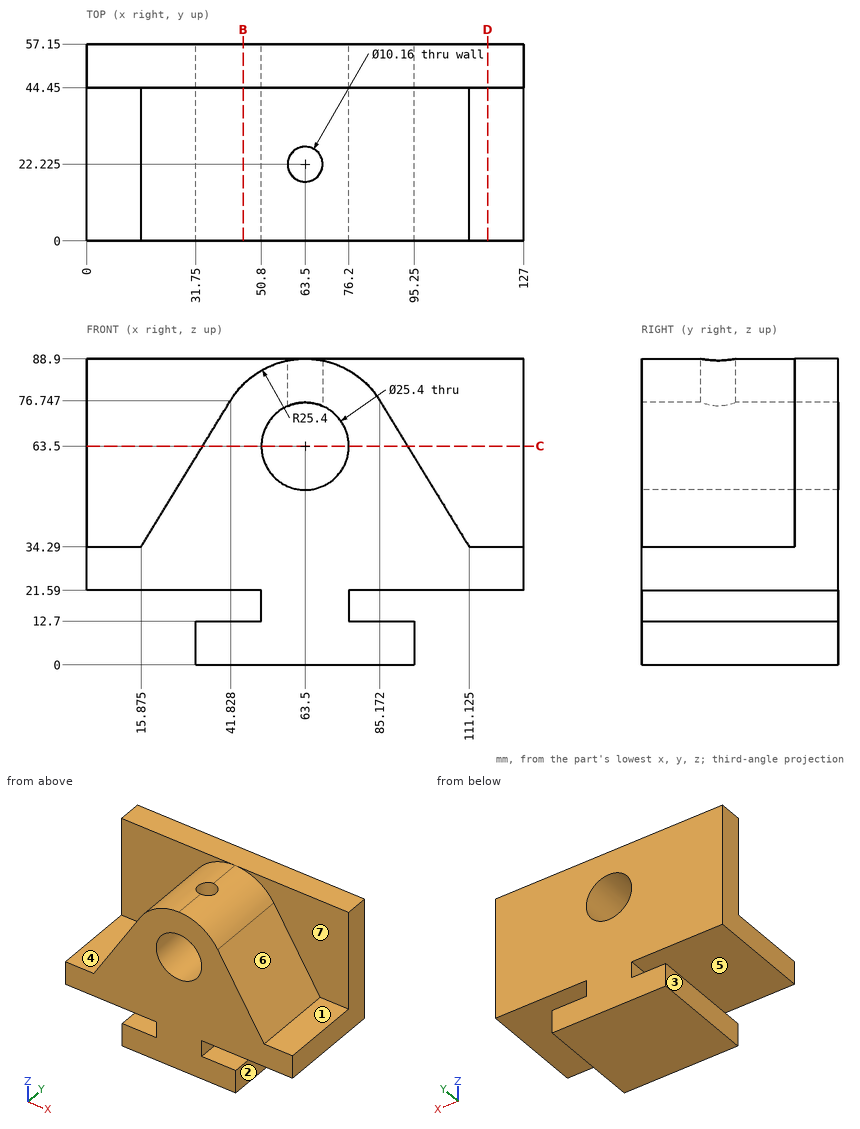
Here's the drawing with two shaded views (mm, measured from the low corner). I have some questions. A direction names the side the tool comes from. Give positions to 0.01 mm unless a question says otherwise; leave off trailing zeros. Loops run counter-clockwise (first coordinate to the right, second up) from the corner with the lowest first, then second, coordinate; pieces in that order, holes last. Notation, with made-up numbers: (64, 1.5) - (103, 1.5) arc R12 cw to (103, 24.5) - close; hole circle Ø4 at (54.5, 50). An arc over 180 degrees is marked (long way). Return JSON: item names as keys, results as strings.
1. I want a section at D-D on x = 116.5. Please give me the cut outline in (y, z), and give its area (3 significant figures).
Output values:
{"outline": "(0, 21.59) - (57.15, 21.59) - (57.15, 88.9) - (44.45, 88.9) - (44.45, 34.29) - (0, 34.29) - close", "area": "1,420 mm²"}
2. For the marked faces 1, 2, 3 and 4, which set-ups out of +Z, -Z, +X, -X, +Y, -Y let a thin tool reach every point of the face, with its end or its side?
Output values:
{"face 1": "+Z, +X, -Y", "face 2": "-Z, +X, +Y, -Y", "face 3": "-Z, -X, +Y, -Y", "face 4": "+Z, -X, -Y"}
3. If I drill on line 1 (Z direction, x = 63.5, y = 42); line 2 (Z direction, x = 87, y = 53.5); line 3 (X direction, y = 43.5, z = 17), over which ranges is the centre line in solid material (lowest first)?
Output values:
{"line 1": "z = 0 to 50.8, 76.2 to 88.9", "line 2": "z = 0 to 12.7, 21.59 to 88.9", "line 3": "x = 50.8 to 76.2"}
4. I want a section at B-B on x = 45.5. Please give me the cut outline in (y, z).
Output values:
{"outline": "(0, 0) - (57.15, 0) - (57.15, 12.7) - (0, 12.7) - close; (0, 21.59) - (57.15, 21.59) - (57.15, 88.9) - (44.45, 88.9) - (44.45, 81.42) - (0, 81.42) - close"}
5. I'm going to push flat-ended pins straight in: pin 1 Ø9.5 at (x, y) = (39, 29) entering from +Z; pin 2 Ø5 at (x, y) = (122.5, 32) entering from +Z; pin 3 Ø2.5 at (y, z) = (22, 18.5) entering from -X. Where does each tip first touch, or does it pass through?
Output values:
{"pin 1": "stops at z = 79.47", "pin 2": "stops at z = 34.29", "pin 3": "stops at x = 50.8"}
6. We'd pull the mould along Z, two halves only. Please class the marked faces 5, 6 and 7: +Z half, -Z half, draft (parallel to the pull), parting line (faces both ways), or undercut.
Output values:
{"face 5": "undercut", "face 6": "+Z half", "face 7": "draft"}
7. I want a section at C-C on z = 63.5. Please give me the cut outline in (x, y).
Output values:
{"outline": "(0, 44.45) - (33.73, 44.45) - (33.73, 0) - (50.8, 0) - (50.8, 57.15) - (0, 57.15) - close; (76.2, 0) - (93.27, 0) - (93.27, 44.45) - (127, 44.45) - (127, 57.15) - (76.2, 57.15) - close"}
